Check sheet for the modelled part. Datum: model origin and axes. Units: mm. A direction names the side the tool comes from. Coordinates: 2 decimals unless noted, no trailing zeros. Loops run counter-clockwise (first coordinate to the right, second up) from the corner with the lowest first, then second, coordinate; pieces in that order, holes last. Notation, with made-up numbers: (11, 16) -> (27, 16) arc R28 ccw to (27, 47) -> close; hole circle Ø4 at (33.25, 80). An arc over 180 degrees is marked (long way). Use CSV: the item, a comma, the result in double quotes.
```python
from build123d import *

# Parameters (mm, degrees)
SKETCH_1_W          = 31
SKETCH_1_H          = 21
EXTRUDE_1_DEPTH     = 5
SKETCH_2_W          = 31
SKETCH_2_H          = 3
EXTRUDE_2_DEPTH     = 10
SKETCH_5_R          = 1.5
CUT_EXTRUDE_2_DEPTH = 31.103986447
SKETCH_6_R          = 1.5
CUT_EXTRUDE_3_DEPTH = 24.989581072
SKETCH_7_W          = 31
SKETCH_7_H          = 2
EXTRUDE_3_DEPTH     = 2


with BuildPart() as part:
    # 草图1 → 凸台-拉伸1 (new body)
    with BuildSketch(Plane.XY):
        Rectangle(SKETCH_1_W, SKETCH_1_H)
    extrude(amount=EXTRUDE_1_DEPTH)

    # 草图2 → 凸台-拉伸2 (add)
    with BuildSketch(Plane.XY.offset(5)):
        with Locations((0, 9)):
            Rectangle(SKETCH_2_W, SKETCH_2_H)
        with Locations((0, -9)):
            Rectangle(SKETCH_2_W, SKETCH_2_H)
    extrude(amount=EXTRUDE_2_DEPTH)

    # 草图5 → 切除-拉伸2 (cut, through all)
    with BuildSketch(Plane(origin=(0, 10.5, 0), x_dir=(1, 0, 0), z_dir=(0, 1, 0))):
        with Locations(Location((11, -11, 0), (0, 0, 270))):
            Circle(SKETCH_5_R)
        with Locations(Location((-11, -11, 0), (0, 0, 270))):
            Circle(SKETCH_5_R)
    extrude(amount=-CUT_EXTRUDE_2_DEPTH, mode=Mode.SUBTRACT)

    # 草图6 → 切除-拉伸3 (cut, through all)
    with BuildSketch(Plane(origin=(0, 0, 0), x_dir=(-1, 0, 0), z_dir=(0, 0, -1))):
        with Locations((-11, 0)):
            Circle(SKETCH_6_R)
        with Locations(Location((11, 0, 0), (0, 0, 180))):
            Circle(SKETCH_6_R)
    extrude(amount=-CUT_EXTRUDE_3_DEPTH, mode=Mode.SUBTRACT)

    # 草图7 → 凸台-拉伸3 (add)
    with BuildSketch(Plane.XY.offset(5)):
        with Locations((0, -6.5)):
            Rectangle(SKETCH_7_W, SKETCH_7_H)
        with Locations((0, 6.5)):
            Rectangle(SKETCH_7_W, SKETCH_7_H)
    extrude(amount=EXTRUDE_3_DEPTH)


solid = part.part
```
1) Cross-section at C-C on z = 5.5. Record the boundary of the cut face in (x, y).
Answer below:
outline,"(-15.5, -10.5) -> (15.5, -10.5) -> (15.5, -5.5) -> (-15.5, -5.5) -> close; (-15.5, 5.5) -> (15.5, 5.5) -> (15.5, 10.5) -> (-15.5, 10.5) -> close"
2) Thickness scan on line 1 along X through (y, z) = (-9.4, 11); line 2 along Y through (x, z) = (5, 5.75); line 3 along Y through (x, z) = (3.5, 12.5). Record the ranges inside material, lowest first. Write a range as from..to.
Answer below:
line 1,"x = -15.5..-12.5, -9.5..9.5, 12.5..15.5"
line 2,"y = -10.5..-5.5, 5.5..10.5"
line 3,"y = -10.5..-7.5, 7.5..10.5"
3) Go/stop test with flat-tipped pins: pin 1 Ø2 at (y, z) = (5.5, 9.5) entering from -X; pin 2 Ø0.6 at (x, y) = (7.5, 6.5) entering from +Z; pin 3 Ø3.5 at (x, y) = (6.5, -1.5) entering from +Z. Record where each tip stops, or that it passes through.
Answer below:
pin 1,"passes through"
pin 2,"stops at z = 7"
pin 3,"stops at z = 5"
4) Cross-section at A-A on y = 0. Record the boundary of the cut face in (x, z).
Answer below:
outline,"(-15.5, 0) -> (-12.5, 0) -> (-12.5, 5) -> (-15.5, 5) -> close; (-9.5, 0) -> (9.5, 0) -> (9.5, 5) -> (-9.5, 5) -> close; (12.5, 0) -> (15.5, 0) -> (15.5, 5) -> (12.5, 5) -> close"
5) Cross-section at D-D on z = 11.5. Record the boundary of the cut face in (x, y), and give its area (3 significant figures).
Answer below:
outline,"(-15.5, -10.5) -> (-12.41, -10.5) -> (-12.41, -7.5) -> (-15.5, -7.5) -> close; (-15.5, 7.5) -> (-12.41, 7.5) -> (-12.41, 10.5) -> (-15.5, 10.5) -> close; (-9.59, -10.5) -> (9.59, -10.5) -> (9.59, -7.5) -> (-9.59, -7.5) -> close; (-9.59, 7.5) -> (9.59, 7.5) -> (9.59, 10.5) -> (-9.59, 10.5) -> close; (12.41, -10.5) -> (15.5, -10.5) -> (15.5, -7.5) -> (12.41, -7.5) -> close; (12.41, 7.5) -> (15.5, 7.5) -> (15.5, 10.5) -> (12.41, 10.5) -> close"
area,"152 mm²"
6) Cross-section at B-B on x = -11. Record the boundary of the cut face in (y, z), and give its area (3 significant figures).
Answer below:
outline,"(-10.5, 0) -> (-1.5, 0) -> (-1.5, 5) -> (-5.5, 5) -> (-5.5, 7) -> (-7.5, 7) -> (-7.5, 9.5) -> (-10.5, 9.5) -> close; (-10.5, 12.5) -> (-7.5, 12.5) -> (-7.5, 15) -> (-10.5, 15) -> close; (1.5, 0) -> (10.5, 0) -> (10.5, 9.5) -> (7.5, 9.5) -> (7.5, 7) -> (5.5, 7) -> (5.5, 5) -> (1.5, 5) -> close; (7.5, 12.5) -> (10.5, 12.5) -> (10.5, 15) -> (7.5, 15) -> close"
area,"140 mm²"
7) Draft check along X on faces 3 (the flat face through (0, 7.5, 11)), 4 (the flat face through (-15.5, 0, 4)), 5 (the cylindrical face through (12.5, 0.07, 2.46)). Enter one of: released by +X, released by -X, zero draft, split by the parting line, or undercut.
Answer below:
face 3,"zero draft"
face 4,"released by -X"
face 5,"undercut"
8) Access from +Z, -Z, +X, -X, +Y, -Y to the whole of each face (thin tool, end or side, straight path). Record for faces 1 (the flat face through (0, 9, 15)), 2 (the flat face through (0, 0, 5)).
Answer below:
face 1,"+Z, +X, -X, +Y, -Y"
face 2,"+Z, +X, -X"
